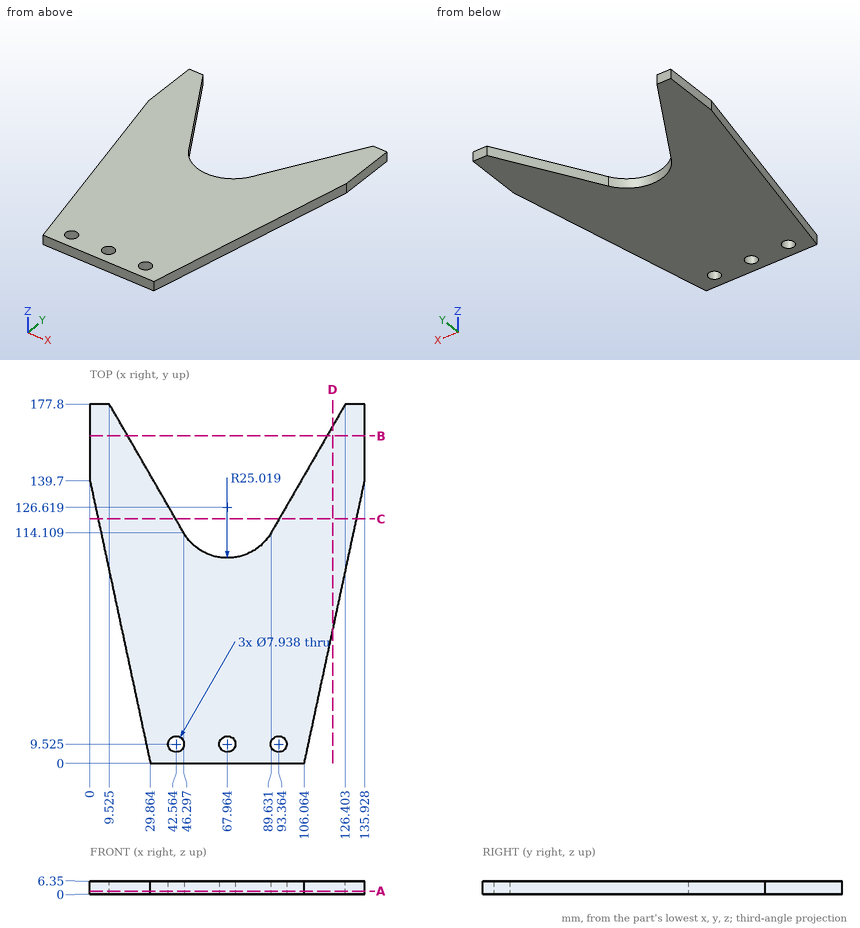
Job drawing, mm, ordinate dimensions from the low corner. One solid piece. Round coordinates to 2 decimals unless told otherwise and drop trailing zeros. Loops run counter-clockwise (first coordinate to the right, second up) from the corner with the lowest first, then second, coordinate; pieces in that order, holes last. Notation, with made-up numbers: (-5.75, 53.25) -> (34.25, 53.25) arc R22 ccw to (34.25, 80.25) -> close; hole circle Ø6 at (49, -31). An arc over 180 degrees is marked (long way). One line per item, written item: value. Start each with the question number.
Q1. Cut at D-D on x = 120. List the corners of the cut face in (y, z).
Q2. Cut at B-B on y = 162. List the corners of the cut face in (x, z), plus the area to 3 significant figures.
Q3. Probe line 1 along X through (y, z) = (8, 5.25) (1 decimal); line 2 along X through (y, z) = (9.5, 4.25) (1 decimal); line 3 along X through (y, z) = (117.5, 3.5) (1 decimal). List the from-to ranges inside material, lowest first.
Q4. Drop flat-ended pins along their axis: pin 1 Ø8 at (x, y) = (42, 98.5) entering from -Z; pin 2 Ø3 at (y, z) = (36.5, 4) entering from +X; pin 3 Ø6.5 at (x, y) = (93.36, 9.53) entering from +Z; pin 4 Ø1 at (y, z) = (118.5, 2) entering from +X. Give the stop position or say it passes through.
Q5. Cut at A-A on z = 1.5. List the corners of the cut face in (x, y) (1 decimal), plus the area to 3 significant figures.
Q6. Cut at C-C on y = 121. List the corners of the cut face in (x, z).
Computed:
1. outline: (65.19, 0) -> (166.71, 0) -> (166.71, 6.35) -> (65.19, 6.35) -> close
2. outline: (0, 0) -> (18.65, 0) -> (18.65, 6.35) -> (0, 6.35) -> close; (117.28, 0) -> (135.93, 0) -> (135.93, 6.35) -> (117.28, 6.35) -> close
2. area: 237 mm²
3. line 1: 28.2 to 38.9, 46.2 to 64.3, 71.6 to 89.7, 97 to 107.8
3. line 2: 27.8 to 38.6, 46.5 to 64, 71.9 to 89.4, 97.3 to 108.1
3. line 3: 4.7 to 44.3, 91.6 to 131.2
4. pin 1: z = 0
4. pin 2: x = 114.19
4. pin 3: through
4. pin 4: x = 131.5
5. outline: (0, 139.7) -> (29.9, 0) -> (106.1, 0) -> (135.9, 139.7) -> (135.9, 177.8) -> (126.4, 177.8) -> (89.6, 114.1) arc R25 cw to (46.3, 114.1) -> (9.5, 177.8) -> (0, 177.8) -> close; hole circle Ø7.9 at (42.6, 9.5); hole circle Ø7.9 at (68, 9.5); hole circle Ø7.9 at (93.4, 9.5)
5. area: 14,400 mm²
6. outline: (4, 0) -> (42.32, 0) -> (42.32, 6.35) -> (4, 6.35) -> close; (93.61, 0) -> (131.93, 0) -> (131.93, 6.35) -> (93.61, 6.35) -> close
